Read the model definition and answer for the solid it produces. Units are mm, in the model's axes. Face numbers are marked on the shaded views. A direction names the side the tool comes from. Round coordinates to 2 decimals unless told otherwise and drop trailing zeros. Order: outer loops, then holes, each group sorted by start corner. A loop starts at its lowest first (then second) coordinate and runs counter-clockwise, first axis right, second up. Notation, with made-up numbers: (71.5, -26) - (79.5, -26) arc R8 cw to (79.5, -16) - close; hole circle Ø4 at (80.5, 25.5). An arc over 180 degrees is marked (long way). Put each result on its own line as item: value. Start each with the question number.
Q1. Each of these flat-tipped pins is pushed along its axis until it touches: pin 1 Ø1 at (y, z) = (0.5, 2) entering from -X; pin 2 Ø8 at (x, z) = (-1, -1) entering from -Y; pin 3 Ø5 at (x, z) = (-3, 1) entering from -Y. Where does it stop, or does it pass through?
Q2. Section D-D on y = 6.5 is taken. Give the vertices of the cut face in (x, z).
Q3. Find the intervals of material crossed by line 1 along Y through (x, z) = (3.75, 5.5); line 2 along X through (y, z) = (8.5, 0.25); line 3 along X through (y, z) = (9, -2.75), in increasing order. Write a range as from..to.
Q4. Section C-C on y = -0.5 is taken. Give the vertices of the cut face in (x, z).
Q5. Which of the six approach directions +Z, -Z, +X, -X, +Y, -Y give full straight-line access (tool end or side, diameter ignored) to the marked faces 1, 2 and 3?
from build123d import *

# Parameters (mm, degrees)
F0_R     = 7.5
F1_DEPTH = 15
F2_R     = 9
F3_DEPTH = 2
F4_R     = 6
F5_DEPTH = 2
F7_DEPTH = 12.5
F8_R     = 1.99999


# Not quite as in the source:
# - a fillet or chamfer is up to 0.001 mm smaller than in the source, because OpenCascade refuses the exact size


with BuildPart() as f1:
    # F0 (on Front) → F1 (new body)
    with BuildSketch(Plane.XZ):
        Circle(F0_R)
    extrude(amount=-F1_DEPTH)

    # F2 (on Front) → F3 (join)
    with BuildSketch(Plane.XZ):
        Circle(F2_R)
    extrude(amount=-F3_DEPTH)

    # F4 (on Front) → F5 (join)
    with BuildSketch(Plane.XZ):
        Circle(F4_R)
    extrude(amount=F5_DEPTH)

    # F6 (on Right) → F7 (cut, symmetric)
    with BuildSketch(Plane.YZ):
        with BuildLine():
            ThreePointArc((-2, -6), (-1.1103724444, 0), (-2, 6))
            Line((-2, 6), (-2, -6))
        make_face()
    extrude(amount=F7_DEPTH, both=True, mode=Mode.SUBTRACT)

    # F8 (radius 2 in the source; OpenCascade refuses exactly that, so slightly less here)
    f8_edges = [f1.edges().sort_by_distance(p)[0] for p in [
        (-9, 0, 0),
    ]]
    fillet(f8_edges, radius=F8_R)


solid = f1.part
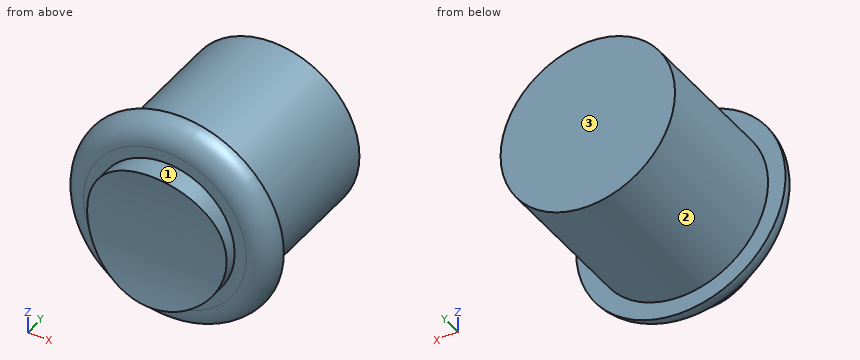
Findings:
1. pin 1: x = -8.52
1. pin 2: y = -1.72
1. pin 3: y = -1.41
2. outline: circle Ø15 at (0, 0)
3. line 1: 0..15
3. line 2: -7.5..7.5
3. line 3: -6.98..6.98
4. outline: circle Ø12 at (0, 0)
5. face 1: -Y
5. face 2: +Y
5. face 3: +Z, -Z, +X, -X, +Y
